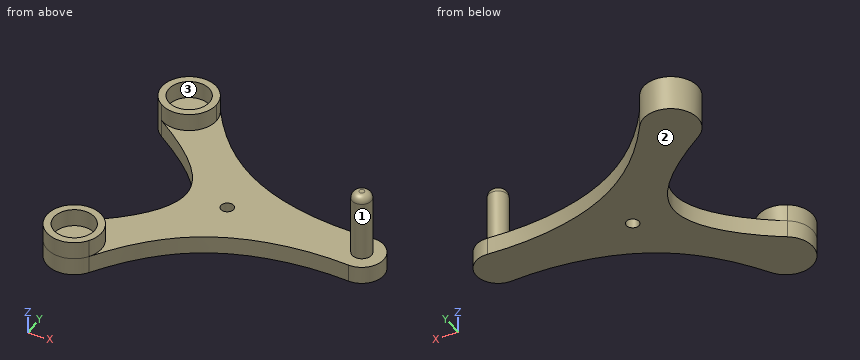
```python
from build123d import *

# Parameters (mm, degrees)
F0_R     = 1.8
F0_R_2   = 2.75
F0_R_3   = 5.75
F1_DEPTH = 5
F2_DEPTH = 5
F3_DEPTH = 19
F4_R     = 2


with BuildPart() as f1:
    # F0 (on Top) → F1 (new body)
    with BuildSketch(Plane.XY):
        with BuildLine():
            ThreePointArc((-20.5278924674, 33.9874824942), (-19.5887790687, 31.9605740028), (-19.2668247456, 29.75))
            ThreePointArc((-19.2668247456, 29.75), (-23.4010274534, 22.8951834494), (-31.3928918273, 23.3537091298))
            add(Edge.make_bspline(
                [(-31.3928918273, 23.3537091298), (-21.6948142815, 16.7187016285), (-1.5034517677, 0.3606813033), (-21.4654354866, -17.2386169061), (-31.0762132171, -23.1481922751)],
                knots=[0, 0, 0, 0, 0.5014830117, 1, 1, 1, 1], degree=3))
            ThreePointArc((-31.0762132171, -23.1481922751), (-23.2351426235, -22.9852841651), (-19.2668247456, -29.75))
            ThreePointArc((-19.2668247456, -29.75), (-19.5887790687, -31.9605740028), (-20.5278924674, -33.9874824942))
            add(Edge.make_bspline(
                [(-20.5278924674, -33.9874824942), (-14.2038261776, -24.3033273542), (0.8934932617, -9.0476289983), (25.586991994, -5.4412595008), (37.5868020457, -6.2363264387)],
                knots=[0, 0, 0, 0, 0.4873954252, 1, 1, 1, 1], degree=3))
            ThreePointArc((37.5868020457, -6.2363264387), (44.25, 0), (37.5868020457, 6.2363264387))
            add(Edge.make_bspline(
                [(-20.5278924674, 33.9874824942), (-14.2038261776, 24.3033273542), (0.8934932617, 9.0476289983), (25.586991994, 5.4412595008), (37.5868020457, 6.2363264387)],
                knots=[0, 0, 0, 0, 0.4873954252, 1, 1, 1, 1], degree=3))
        make_face()
        Circle(F0_R, mode=Mode.SUBTRACT)
        with Locations((38, 0)):
            Circle(F0_R_2, mode=Mode.SUBTRACT)
        with BuildLine():
            ThreePointArc((-31.3928918273, 23.3537091298), (-23.4010274534, 22.8951834494), (-19.2668247456, 29.75))
            ThreePointArc((-19.2668247456, 29.75), (-19.5887790687, 31.9605740028), (-20.5278924674, 33.9874824942))
            ThreePointArc((-20.5278924674, 33.9874824942), (-32.4376488366, 35.2886971549), (-31.3928918273, 23.3537091298))
        make_face()
        with Locations((-27.0168247456, 29.75)):
            Circle(F0_R_3, mode=Mode.SUBTRACT)
        with BuildLine():
            ThreePointArc((-19.2668247456, -29.75), (-23.2351426235, -22.9852841651), (-31.0762132171, -23.1481922751))
            ThreePointArc((-31.0762132171, -23.1481922751), (-32.5709424875, -35.1550232293), (-20.5278924674, -33.9874824942))
            ThreePointArc((-20.5278924674, -33.9874824942), (-19.5887790687, -31.9605740028), (-19.2668247456, -29.75))
        make_face()
        with Locations((-27.0168247456, -29.75)):
            Circle(F0_R_3, mode=Mode.SUBTRACT)
        with Locations((-27.0168247456, 29.75)):
            Circle(F0_R_3)
        with Locations((-27.0168247456, -29.75)):
            Circle(F0_R_3)
        with Locations((38, 0)):
            Circle(F0_R_2)
    extrude(amount=-F1_DEPTH)

    # F0 (on Top) → F2 (join)
    with BuildSketch(Plane.XY):
        with BuildLine():
            ThreePointArc((-31.3928918273, 23.3537091298), (-23.4010274534, 22.8951834494), (-19.2668247456, 29.75))
            ThreePointArc((-19.2668247456, 29.75), (-19.5887790687, 31.9605740028), (-20.5278924674, 33.9874824942))
            ThreePointArc((-20.5278924674, 33.9874824942), (-32.4376488366, 35.2886971549), (-31.3928918273, 23.3537091298))
        make_face()
        with Locations((-27.0168247456, 29.75)):
            Circle(F0_R_3, mode=Mode.SUBTRACT)
        with BuildLine():
            ThreePointArc((-19.2668247456, -29.75), (-23.2351426235, -22.9852841651), (-31.0762132171, -23.1481922751))
            ThreePointArc((-31.0762132171, -23.1481922751), (-32.5709424875, -35.1550232293), (-20.5278924674, -33.9874824942))
            ThreePointArc((-20.5278924674, -33.9874824942), (-19.5887790687, -31.9605740028), (-19.2668247456, -29.75))
        make_face()
        with Locations((-27.0168247456, -29.75)):
            Circle(F0_R_3, mode=Mode.SUBTRACT)
    extrude(amount=F2_DEPTH)

    # F0 (on Top) → F3 (join)
    with BuildSketch(Plane.XY):
        with Locations((38, 0)):
            Circle(F0_R_2)
    extrude(amount=F3_DEPTH)

    # F4
    f4_edges = [f1.edges().sort_by_distance(p)[0] for p in [
        (35.25, 0, 19),
    ]]
    fillet(f4_edges, radius=F4_R)


solid = f1.part
```
Verification items for the finished model (mm, model axes). Face numbers are marked on the shaded views. Coordinates: 2 decimals unless noted, no trailing zeros. Write each loop counter-clockwise with the first axis right and the second up, starting at its lowest first coordinate (ties: lowest second). Pieces come first, ordered by that corner, then holes. Notation, with made-up numbers: M 82.25,82.5 L 119.25,82.5 A19 cw 119.25,93.5 Z; hole C 81,87.25 d10. An arc over 180 degrees is marked long. Answer as a JSON object with one key per item and string values. Group by question number.
(1) Cross-section at A-A, the plane z = 12.75. Record the cut outline in (x, y), and give its area (3 significant figures).
(2) Release check for a two-part mould opening along X. For the marked faces 1, 2 and 3 record: +X half, -X half, draft (parallel to the pull), parting line (faces both ways), or undercut.
(3) Gauge pin test, flat ends, axial feed: pin 1 (1.5 mm diameter, centred on x = -18, y = -12, fed in from +Z); pin 2 (12.5 mm diameter, centred on x = -29.5, y = 32, fed in from +Z); pin 3 (5 mm diameter, centred on x = -6, z = 1.5, fed in from +Y). Record the tip position at first contact, or that the pin passes through.
(4) Material ranges on line 1 (Y direction, x = -26.5, z = 2.5); line 2 (Z direction, x = -18.5, y = -14.5); line 3 (Z direction, x = -26.5, y = -23.5), recorded low to high.
Reply:
{
 "1": {"outline": "C 38,0 d5.5", "area": "23.8 mm²"},
 "2": {"face 1": "parting line", "face 2": "draft", "face 3": "undercut"},
 "3": {"pin 1": "z = 0", "pin 2": "z = 5", "pin 3": "y = 19.3"},
 "4": {"line 1": "-37.48 to -35.48, -24.02 to -22.02, 22.02 to 24.02, 35.48 to 37.48", "line 2": "-5 to 0", "line 3": "-5 to 5"}
}
